from build123d import *

# Parameters (mm, degrees)
SKETCH1_R           = 1.5875
BOSS_EXTRUDE1_DEPTH = 19.05
SKETCH2_R           = 2.2225
BOSS_EXTRUDE2_DEPTH = 3.175
MOVE_FACE1_BY       = 0.250000008


with BuildPart() as part:
    # Sketch1 → Boss-Extrude1 (new body)
    with BuildSketch(Plane.XY):
        with Locations(Location((0, 0, 0), (0, 0, 180))):
            Circle(SKETCH1_R)
    extrude(amount=BOSS_EXTRUDE1_DEPTH)

    # Sketch2 → Boss-Extrude2 (add)
    with BuildSketch(Plane.XY.offset(19.05)):
        Circle(SKETCH2_R)
    extrude(amount=BOSS_EXTRUDE2_DEPTH)

    # Move Face1: a curved face moved inward by 0.25
    add(Solid.thicken(part.faces().sort_by_distance((1.5875, 0, 9.525))[0], -MOVE_FACE1_BY), mode=Mode.SUBTRACT)


solid = part.part
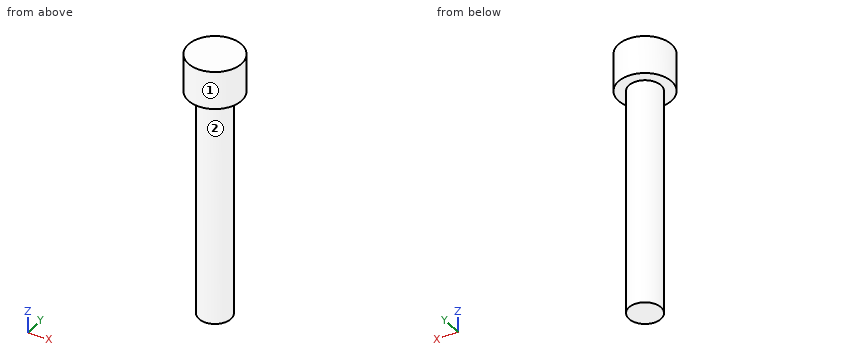
Geometry: final body of the model. Coordinates: model frame, mm. Face numbers are marked on the shaded views. A direction names the side the tool comes from. Coordinates: 2 decimals unless noted, no trailing zeros. Order: outer loops, then holes, each group sorted by start corner. A loop starts at its lowest first (then second) coordinate and runs counter-clockwise, first axis right, second up.
(1) Section query C-C (z = 10.25). Return the cut outline in (x, y) (1 decimal), plus the area to 3 significant figures.
(2) Section query B-B (x = 0.55). Return the cut outline in (y, z) (3 decimals), plus the area to 3 significant figures.
(3) First-contact query: pin 1 (2 mm diameter, centred on y = -1, z = 10.5, fed in from -X). Flat tip, straight axial feed; report the tip coordinate or a pass-through.
(4) Access query for the marked faces 1 and 2. Directions: +Z, -Z, +X, -X, +Y, -Y. A direction counts if a zero-diameter tool reaches every point of the face in a straight line with its end or side. Return the directions, or none.
(5) Material intervals for probe 1 along Z at (x, y) = (1.95, 0.45) (3 decimals); probe 2 along Y at (x, z) = (0.1, 4.75); probe 3 along X at (y, z) = (-0.4, 7), sorted ascending.
Solution:
1. outline: circle Ø2.7 at (0, 0)
1. area: 5.62 mm2
2. outline: (-2.153, 19.05) - (-1.219, 19.05) - (-1.219, 0) - (1.219, 0) - (1.219, 19.05) - (2.153, 19.05) - (2.153, 22.225) - (-2.153, 22.225) - close
2. area: 60.1 mm2
3. pin 1: stops at x = -1.34
4. face 1: +Z, -Z
4. face 2: -Z
5. probe 1: z = 19.05 to 22.225
5. probe 2: y = -1.33 to 1.33
5. probe 3: x = -1.28 to 1.28
